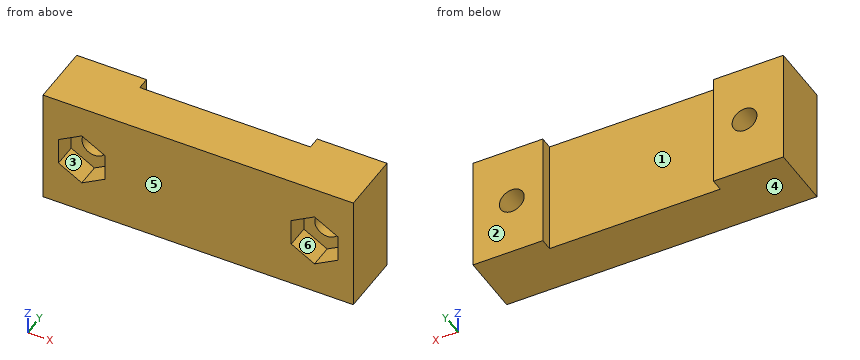
from build123d import *

# Parameters (mm, degrees)
SKETCH1_W           = 40
SKETCH1_H           = 15
BOSS_EXTRUDE1_DEPTH = 8
SKETCH2_R           = 1.6
CUT_EXTRUDE1_DEPTH  = 23.808989456
SKETCH3_W           = 22
SKETCH3_H           = 15
CUT_EXTRUDE2_DEPTH  = 1.6
CUT_EXTRUDE3_DEPTH  = 3


with BuildPart() as part:
    # Sketch1 → Boss-Extrude1 (new body)
    with BuildSketch(Plane(origin=(0, 0, 0), x_dir=(1, 0, 0), z_dir=(0, 1, 0))):
        Rectangle(SKETCH1_W, SKETCH1_H)
    extrude(amount=BOSS_EXTRUDE1_DEPTH)

    # Sketch2 → Cut-Extrude1 (cut, through all)
    with BuildSketch(Plane(origin=(0, 8, 0), x_dir=(1, 0, 0), z_dir=(0, 1, 0))):
        with Locations(Location((-15, 0, 0), (0, 0, 270))):
            Circle(SKETCH2_R)
        with Locations(Location((15, 0, 0), (0, 0, 270))):
            Circle(SKETCH2_R)
    extrude(amount=-CUT_EXTRUDE1_DEPTH, mode=Mode.SUBTRACT)

    # Sketch3 → Cut-Extrude2 (cut)
    with BuildSketch(Plane(origin=(0, 8, 0), x_dir=(1, 0, 0), z_dir=(0, 1, 0))):
        Rectangle(SKETCH3_W, SKETCH3_H)
    extrude(amount=-CUT_EXTRUDE2_DEPTH, mode=Mode.SUBTRACT)

    # Sketch4 → Cut-Extrude3 (cut)
    with BuildSketch(Plane.XZ):
        Polygon((-12, 1.732050808), (-15, 3.464101615), (-18, 1.732050808), (-18, -1.732050808), (-15, -3.464101615), (-12, -1.732050808), align=None)
        Polygon((12, -1.732050808), (12, 1.732050808), (15, 3.464101615), (18, 1.732050808), (18, -1.732050808), (15, -3.464101615), align=None)
    extrude(amount=-CUT_EXTRUDE3_DEPTH, mode=Mode.SUBTRACT)


solid = part.part
Geometry check sheet. Reference: the model listing, model coordinates, mm. Face numbers are marked on the shaded views. A direction names the side the tool comes from. Coordinates: 2 decimals unless noted, no trailing zeros. Order: outer loops, then holes, each group sorted by start corner. A loop starts at its lowest first (then second) coordinate and runs counter-clockwise, first axis right, second up. Notation, with made-up numbers: (70, -13) - (92, -13) arc R16 cw to (92, -3) - close; hole circle Ø2 at (53, 73.5). An arc over 180 degrees is marked (long way). Answer in a Markdown table with one row per item. Add a question column.
1) Set-up check for the marked faces 1, 2 and 3: record each of +Z, -Z, +X, -X, +Y, -Y from which the full face is reachable in a straight line by a thin tool's end or side.
2) Cross-section at C-C, the plane y = 2. Record the cut outline in (x, z).
3) Material ranges on line 1 along X through (y, z) = (6.6, 0); line 2 along X through (y, z) = (5.1, 0); line 3 along X through (y, z) = (2.5, 0.5), recorded low to high. Write a range as [from, to].
4) Gauge pin test, flat ends, axial feed: P1, Ø1.9, axis at x = -15, z = 0, coming from the -Y side; P2, Ø3, axis at x = 14.5, z = -0.5, coming from the -Y side; P3, Ø4, axis at x = -1.5, z = -1, coming from the +Y side. Record the tip position at first contact, or that the pin passes through.
5) Cross-section at B-B, the plane z = 0. Record the cut outline in (x, y).
6) Cross-section at D-D, the plane x = 16. Record the cut outline in (y, z).
7) Release check for a two-part mould opening along Z. For the marked faces 4, 5 and 6 record: +Z half, -Z half, draft (parallel to the pull), parting line (faces both ways), or undercut.
8) Cross-section at A-A, the plane y = 7.25. Record the cut outline in (x, z), then the cut area to 3 significant figures.
Check result:
| question | item | result |
|---|---|---|
| 1 | face 1 | +Z, -Z, +Y |
| 1 | face 2 | +Z, -Z, +X, -X, +Y |
| 1 | face 3 | -Y |
| 2 | outline | (-20, -7.5) - (20, -7.5) - (20, 7.5) - (-20, 7.5) - close; hole (-18, -1.73) - (-15, -3.46) - (-12, -1.73) - (-12, 1.73) - (-15, 3.46) - (-18, 1.73) - close; hole (12, -1.73) - (15, -3.46) - (18, -1.73) - (18, 1.73) - (15, 3.46) - (12, 1.73) - close |
| 3 | line 1 | x = [-20, -16.6], [-13.4, -11], [11, 13.4], [16.6, 20] |
| 3 | line 2 | x = [-20, -16.6], [-13.4, 13.4], [16.6, 20] |
| 3 | line 3 | x = [-20, -18], [-12, 12], [18, 20] |
| 4 | P1 | passes through |
| 4 | P2 | stops at y = 3 |
| 4 | P3 | stops at y = 6.4 |
| 5 | outline | (-20, 0) - (-18, 0) - (-18, 3) - (-16.6, 3) - (-16.6, 8) - (-20, 8) - close; (-13.4, 3) - (-12, 3) - (-12, 0) - (12, 0) - (12, 3) - (13.4, 3) - (13.4, 8) - (11, 8) - (11, 6.4) - (-11, 6.4) - (-11, 8) - (-13.4, 8) - close; (16.6, 3) - (18, 3) - (18, 0) - (20, 0) - (20, 8) - (16.6, 8) - close |
| 6 | outline | (0, -7.5) - (8, -7.5) - (8, -1.25) - (3, -1.25) - (3, -2.89) - (0, -2.89) - close; (0, 2.89) - (3, 2.89) - (3, 1.25) - (8, 1.25) - (8, 7.5) - (0, 7.5) - close |
| 7 | face 4 | -Z half |
| 7 | face 5 | draft |
| 7 | face 6 | undercut |
| 8 | outline | (-20, -7.5) - (-11, -7.5) - (-11, 7.5) - (-20, 7.5) - close; (11, -7.5) - (20, -7.5) - (20, 7.5) - (11, 7.5) - close; hole circle Ø3.2 at (-15, 0); hole circle Ø3.2 at (15, 0) |
| 8 | area | 254 mm² |
